```python
from build123d import *

# Parameters (mm, degrees)
EXTRUDE_1_DEPTH              = 88
HOLE_WIZARD_M4_1_D           = 4.5
HOLE_WIZARD_M4_1_CBORE_D     = 8
HOLE_WIZARD_M4_1_CBORE_DEPTH = 4.4
HOLE_WIZARD_M4_1_2_D         = 3.3
HOLE_WIZARD_M3_1_D           = 2.5
HOLE_WIZARD_M3_1_DEPTH       = 9.5
HOLE_WIZARD_M3_1_TIP         = 0.751075774
SKETCH_8_R                   = 1.75
CUT_EXTRUDE_1_DEPTH          = 5
SKETCH_9_W                   = 0.6
SKETCH_9_H                   = 88
EXTRUDE_2_DEPTH              = 0.05
HOLE_WIZARD_M4_2_D           = 3.3
HOLE_WIZARD_M4_2_DEPTH       = 5
HOLE_WIZARD_M4_2_TIP         = 0.991420021


with BuildPart() as part:
    # 草图1 → 凸台-拉伸1 (new body)
    with BuildSketch(Plane.XY):
        Polygon((-9, 10), (-9, 5), (-74, 5), (-74, 12), (-79, 12), (-79, 5.9), (-79.6, 5.9), (-79.6, 0), (0, 0), (0, 10), (-2, 10), (-2, 8), (-7, 8), (-7, 10), align=None)
    extrude(amount=EXTRUDE_1_DEPTH)

    # Hole Wizard M4 _1 (through all)
    with Locations(Plane(origin=(0, 0, 0), x_dir=(-1, 0, 0), z_dir=(0, -1, 0))):
        with Locations((4.5, -11.5), (4.5, -44), (4.5, -76.5)):
            CounterBoreHole(HOLE_WIZARD_M4_1_D / 2, HOLE_WIZARD_M4_1_CBORE_D / 2, HOLE_WIZARD_M4_1_CBORE_DEPTH)

    # Hole Wizard M4 _1 2 (through all)
    with Locations(Plane(origin=(0, 0, 0), x_dir=(-1, 0, 0), z_dir=(0, -1, 0))):
        with Locations((68.8, -14), (68.8, -22)):
            Hole(HOLE_WIZARD_M4_1_2_D / 2)

    # M3 螺纹孔1
    with Locations(Plane.ZY.offset(79.6)):
        with Locations((11.5, 3), (44, 3), (76.5, 3)):
            Hole(HOLE_WIZARD_M3_1_D / 2, depth=HOLE_WIZARD_M3_1_DEPTH)
            with Locations((0, 0, -(HOLE_WIZARD_M3_1_DEPTH + HOLE_WIZARD_M3_1_TIP / 2))):  # 118° drill point
                Cone(0, HOLE_WIZARD_M3_1_D / 2, HOLE_WIZARD_M3_1_TIP, mode=Mode.SUBTRACT)

    # 草图8 → 切除-拉伸1 (cut)
    with BuildSketch(Plane.ZY.offset(79)):
        with Locations((63, 9.5)):
            Circle(SKETCH_8_R)
    extrude(amount=-CUT_EXTRUDE_1_DEPTH, mode=Mode.SUBTRACT)

    # 草图9 → 凸台-拉伸2 (add)
    with BuildSketch(Plane(origin=(0, 5.9, 0), x_dir=(1, 0, 0), z_dir=(0, 1, 0))):
        with Locations((-79.3, -44)):
            Rectangle(SKETCH_9_W, SKETCH_9_H)
    extrude(amount=EXTRUDE_2_DEPTH)

    # M4 螺纹孔2
    with Locations(Plane(origin=(0, 0, 0), x_dir=(-1, 0, 0), z_dir=(0, -1, 0))):
        with Locations((74.6, -54.141815628), (74.6, -69.141815628)):
            Hole(HOLE_WIZARD_M4_2_D / 2, depth=HOLE_WIZARD_M4_2_DEPTH)
            with Locations((0, 0, -(HOLE_WIZARD_M4_2_DEPTH + HOLE_WIZARD_M4_2_TIP / 2))):  # 118° drill point
                Cone(0, HOLE_WIZARD_M4_2_D / 2, HOLE_WIZARD_M4_2_TIP, mode=Mode.SUBTRACT)


solid = part.part
```
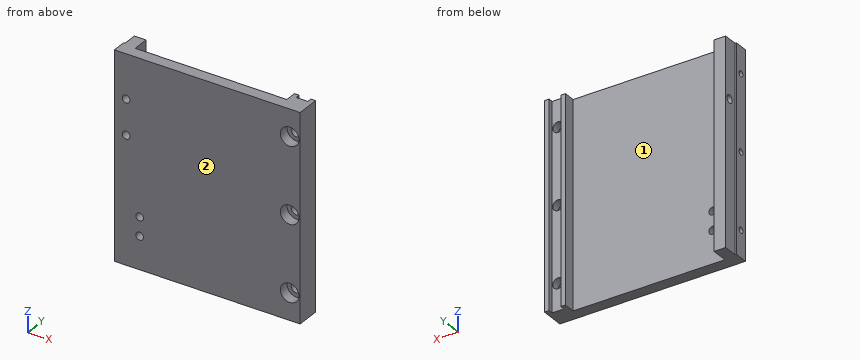
Design review of the part built by this model. Coordinates are the model's own, in mm. Face numbers are marked on the shaded views. Give positions to 0.01 mm unless a question says otherwise; leave off trailing zeros. Order: outer loops, then holes, each group sorted by start corner. A loop starts at its lowest first (then second) coordinate and runs counter-clockwise, first axis right, second up. Notation, with made-up numbers: (27, 82) -> (57, 82) arc R27 cw to (57, 111) -> close; hole circle Ø10 at (44, -10). An arc over 180 degrees is marked (long way). Write each question's results on one line, items separated by ' | '. Start each with the question number.
Q1. Add section B-B on x = -4.5. Give the boundary of the cut face in (y, z).
Q2. Add section C-C on z = 18. Give the boundary of the cut face in (x, y), and give its area (3 significant figures).
Q3. Wall thickness on L1, parallel to Z at x = -68.8, y = 1.75; L2, parallel to Z at x = -4.5, y = 3; L3, parallel to X at y = 8.25, z = 50: over which ranges is each line inside the solid? List them lowest first. Write a range as from..to.
Q4. Add section D-D on x = -66. Give the boundary of the cut face in (y, z), and give its area (3 significant figures).
Q5. Mouldability with a two-part tool opening along X and no side actions: class the marked faces 1 and 2 as +X half, -X half, draft (parallel to the pull), parting line (faces both ways), or undercut.
Q6. Add section A-A on z = 63. Give the boundary of the cut face in (x, y).
Q7. For pin 1 (1.5 mm diameter, centred on y = 3, z = 11.5, fed in from -X); pin 2 (6.5 mm diameter, centred on x = -4, z = 77, fed in from -Y); pin 3 (1.5 mm diameter, centred on x = -14.5, z = 39.5, fed in from +Y), all flat-tipped, find the tip position at first contact; note any pin that passes through.
Found:
1) outline: (0, 0) -> (8, 0) -> (8, 9.25) -> (4.4, 9.25) -> (4.4, 7.5) -> (0, 7.5) -> close; (0, 15.5) -> (4.4, 15.5) -> (4.4, 13.75) -> (8, 13.75) -> (8, 41.75) -> (4.4, 41.75) -> (4.4, 40) -> (0, 40) -> close; (0, 48) -> (4.4, 48) -> (4.4, 46.25) -> (8, 46.25) -> (8, 74.25) -> (4.4, 74.25) -> (4.4, 72.5) -> (0, 72.5) -> close; (0, 80.5) -> (4.4, 80.5) -> (4.4, 78.75) -> (8, 78.75) -> (8, 88) -> (0, 88) -> close
2) outline: (-79.6, 0) -> (0, 0) -> (0, 10) -> (-2, 10) -> (-2, 8) -> (-7, 8) -> (-7, 10) -> (-9, 10) -> (-9, 5) -> (-74, 5) -> (-74, 12) -> (-79, 12) -> (-79, 5.95) -> (-79.6, 5.95) -> close | area: 469 mm2
3) L1: z = 0..12.35, 15.65..20.35, 23.65..88 | L2: z = 0..7.5, 15.5..40, 48..72.5, 80.5..88 | L3: x = -79..-74, -9..-7, -2..0
4) outline: (0, 0) -> (5, 0) -> (5, 88) -> (0, 88) -> close | area: 440 mm2
5) face 1: undercut | face 2: draft
6) outline: (-79.6, 0) -> (0, 0) -> (0, 10) -> (-2, 10) -> (-2, 8) -> (-7, 8) -> (-7, 10) -> (-9, 10) -> (-9, 5) -> (-74, 5) -> (-74, 7.75) -> (-79, 7.75) -> (-79, 5.95) -> (-79.6, 5.95) -> close; (-79, 11.25) -> (-74, 11.25) -> (-74, 12) -> (-79, 12) -> close
7) pin 1: stops at x = -69.8 | pin 2: stops at y = 4.4 | pin 3: stops at y = 5
